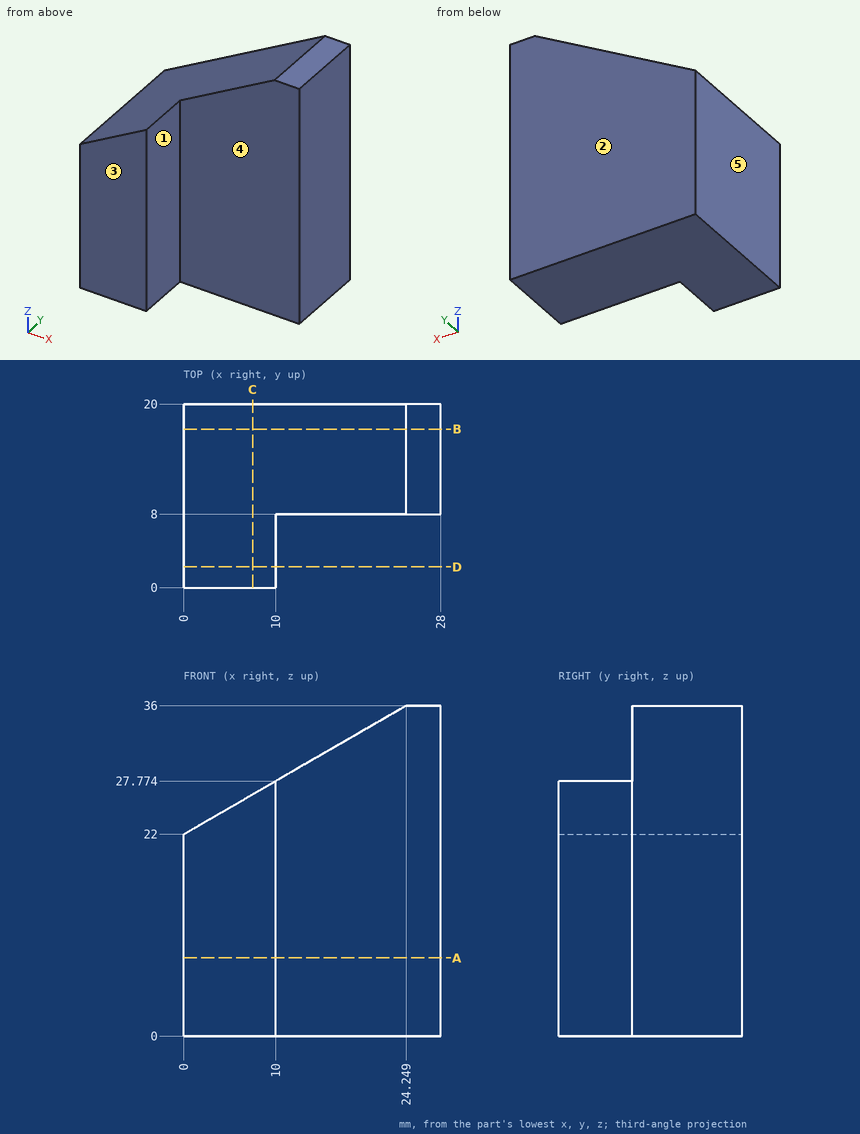
Check sheet for the drawn part. Datum: minimum x, y, z corner. Units: mm. A direction names the side the tool comes from. Give positions to 0.01 mm unless a question says otherwise; leave off trailing zeros. Write each loop counter-clockwise with the first axis right and the second up, starting at its lowest first coordinate (ties: lowest second). Pieces come first, ordered by that corner, then holes. Notation, with made-up numbers: (61.25, -7.75) - (104.25, -7.75) arc R11 ccw to (104.25, 2.25) - close; hole circle Ø10 at (13.5, -14.5). An arc over 180 degrees is marked (long way). Put each result on its own line as item: value.
1. Sectioned sample at D-D, the plane y = 2.25. Enter the section's corners in (x, z).
Ans:
outline: (0, 0) - (10, 0) - (10, 27.77) - (0, 22) - close
2. Set-up check for the marked faces 4 and 5: record each of +Z, -Z, +X, -X, +Y, -Y from which the full face is reachable in a straight line by a thin tool's end or side.
Ans:
face 4: +Z, -Z, +X, -Y
face 5: +Z, -Z, -X, +Y, -Y
3. Sectioned sample at A-A, the plane z = 8.5. Enter the section's corners in (x, y).
Ans:
outline: (0, 0) - (10, 0) - (10, 8) - (28, 8) - (28, 20) - (0, 20) - close
4. Go/stop test with a flat-tipped pin: pin 1 (6 mm diameter, centred on x = 11, z = 32, fed in from -Y). Record where the tip stops, or that it passes through.
Ans:
pin 1: passes through
5. Sectioned sample at C-C, the plane x = 7.5. Enter the section's corners in (y, z), plus the area to 3 significant figures.
Ans:
outline: (0, 0) - (20, 0) - (20, 26.33) - (0, 26.33) - close
area: 527 mm²
6. Thickness scan on line 1 (Y direction, x = 17.5, z = 5); line 2 (Z direction, x = 10, y = 9) (1 decimal); line 3 (X direction, y = 3, z = 20). Record the ranges inside material, lowest first.
Ans:
line 1: y = 8 to 20
line 2: z = 0 to 27.8
line 3: x = 0 to 10
7. Sectioned sample at B-B, the plane y = 17.25. Enter the section's corners in (x, z).
Ans:
outline: (0, 0) - (28, 0) - (28, 36) - (24.25, 36) - (0, 22) - close
8. Draft check along Y on the marked faces 1, 2 and 3. Enter one of: +Y half, -Y half, draft (parallel to the pull), parting line (faces both ways), or undercut.
Ans:
face 1: draft
face 2: +Y half
face 3: -Y half
